Geometry: see drawing. Coordinates: mm, zero at the bounding-box minimum. Give positions to 0.01 mm unless a question says otherwise; leave off trailing zeros. Loops run counter-clockwise (first coordinate to the right, second up) from the corner with the lowest first, then second, coordinate; pieces in that order, holes last. Notation, with made-up numbers: M 67,81 L 118,81 A31 cw 118,108 Z; hole C -5,-34 d8. An arc over 180 degrees is marked long. Return JSON: item names as keys, results as strings. Group by question number.
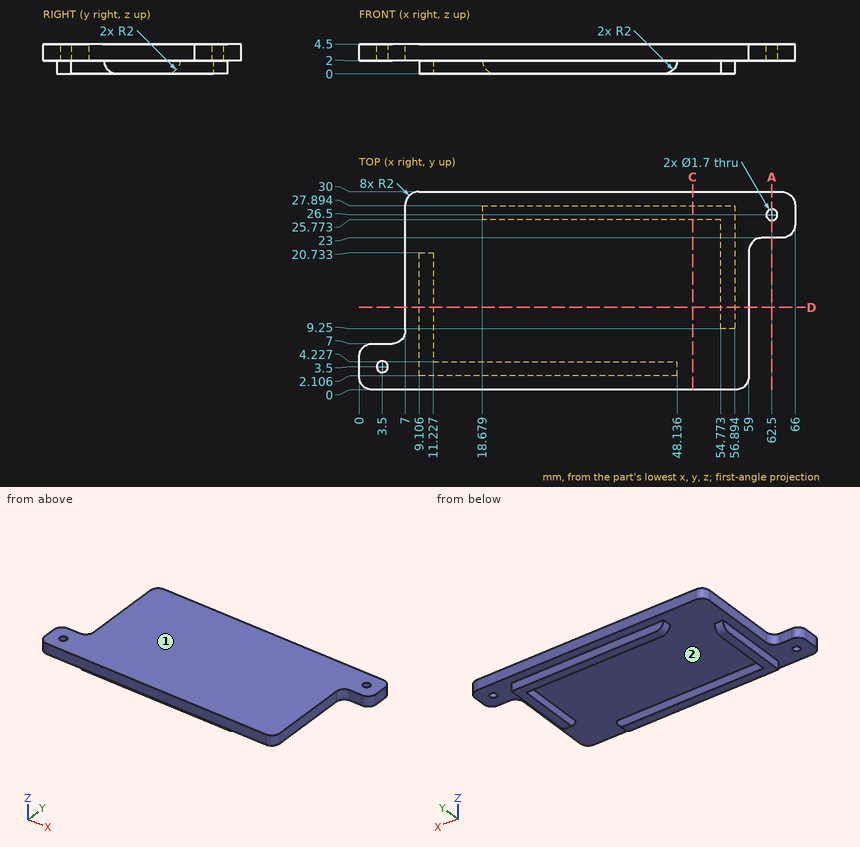
Item 1: Section A-A, the plane x = 62.5. Return loops of the section in (y, z).
Item 2: Section D-D, the plane y = 12.5. Return loops of the section in (x, z) (1 decimal).
Item 3: First-contact query: pin 1 Ø0.6 at (y, z) = (22.5, 1.5) entering from +X; pin 2 Ø0.8 at (y, z) = (13, 3.5) entering from +X; pin 3 Ø0.6 at (x, z) = (37, 1) entering from +Y. Flat tips, straight axial feed; report the tip coordinate or a pass-through.
Item 4: Pull-direction query (X, two-part tool) for the marked faces 1 and 2; classes: pulls with the +X half, pulls with the -X half, needs draft (parallel to the pull), parting line crosses it, or undercut.
Item 5: Material intervals for line 1 (Y direction, x = 62.5, z = 3.45); line 2 (Y direction, x = 45.5, z = 0.7) (1 decimal); line 3 (X direction, y = 19.5, z = 1.85) (1 decimal), sorted ascending. Write a range as from..to.
Item 6: Section C-C, the plane x = 50.5. Return loops of the section in (y, z).
Answer below:
{
 "1": {"outline": "M 23,2 L 25.65,2 L 25.65,4.5 L 23,4.5 Z; M 27.35,2 L 30,2 L 30,4.5 L 27.35,4.5 Z"},
 "2": {"outline": "M 7,2 L 9.1,2 L 9.1,0 L 11.2,0 L 11.2,2 L 54.8,2 L 54.8,0 L 56.9,0 L 56.9,2 L 59,2 L 59,4.5 L 7,4.5 Z"},
 "3": {"pin 1": "x = 56.89", "pin 2": "x = 59", "pin 3": "y = 27.89"},
 "4": {"face 1": "needs draft", "face 2": "undercut"},
 "5": {"line 1": "23..25.65, 27.35..30", "line 2": "2.1..4.2, 25.8..27.9", "line 3": "9.1..11.2, 54.8..56.9"},
 "6": {"outline": "M 0,2 L 25.77,2 L 25.77,0 L 27.89,0 L 27.89,2 L 30,2 L 30,4.5 L 0,4.5 Z"}
}
